Autodesk Inventor part; units mm, degrees
ref_plane "Plano de trabajo1" through (0, 0, 0) normal (0.7071, -0.7071, 0) x (0, 0, 1)
ref_plane "YZ Plane" through (0, 0, 0) normal (1, 0, 0) x (0, 1, 0)
ref_plane "XZ Plane" through (0, 0, 0) normal (0, 1, 0) x (-1, 0, 0)
sketch "Boceto1" plane through (0, 0, 0) normal (0, 0, 1) x (1, 0, 0)
  line L0 (0, 0) -> (0, 25)
  line L1 (0, 0) -> (25, 0)
  line L2 (3, 25) -> (3, 3)
  line L3 (3, 3) -> (25, 3)
  line L4 (0, 25) -> (3, 25)
  line L5 (25, 3) -> (25, 0)
  dimension "d0" = 25
  dimension "d1" = 25
  dimension "d2" = 3
extrude "Extrusión1" add sketch "Boceto1" along normal blind 300
sketch "Boceto2" plane through (0, 0, 0) normal (0, -1, 0) x (1, 0, 0)
  line L0 (0, 0) -> (25, 0) construction
  line L1 (25, 0) -> (25, 300) construction
  line L2 (0, 300) -> (25, 300) construction
  line L3 (0, 0) -> (0, 300) construction
  line L4 (25, 0) -> (25, 300) construction
  line L5 (25, 150) -> (0, 150) construction
  line L6 (25, 300) -> (3, 300)
  line L7 (9, 300) -> (9, 0) construction
  circle A0 centre (9, 159) radius 1.6
  circle A1 centre (9, 141) radius 1.6
  circle A2 centre (9, 279) radius 1.6
  circle A3 centre (9, 261) radius 1.6
  line L8 (25, 270) -> (0, 270) construction
  line L9 (0, 0) -> (0, 300) construction
  dimension "d5" = 3.2
  dimension "d6" = 3.2
  dimension "d7" = 18
  dimension "d8" = 9
  dimension "d9" = 3.2
  dimension "d10" = 3.2
  dimension "d11" = 18
  dimension "d12" = 9
  dimension "d13" = 30
  dimension "d14" = 9
extrude "Extrusión2" cut sketch "Boceto2" against normal through all
ref_plane "Plano de trabajo1" through (0, 0, 0) normal (0.7071, -0.7071, 0) x (0, 0, 1)
mirror "Simetría1" about plane through (0, 0, 0) normal (0.7071, -0.7071, 0) of "Extrusión2"
sketch "Boceto3" plane through (3, 3, 0) normal (0, 1, 0) x (1, 0, 0)
  circle A0 centre (6, -279) radius 1.6 construction
  circle A1 centre (6, -141) radius 1.6 construction
  circle A2 centre (6, -159) radius 1.6 construction
  circle A3 centre (6, -261) radius 1.6 construction
  line L0 (22, 0) -> (0, 0) construction
  line L1 (0, 0) -> (0, -300) construction
  line L2 (22, -300) -> (0, -300) construction
  line L3 (22, 0) -> (22, -300) construction
  circle A4 centre (6, -141) radius 1.6
  circle A5 centre (6, -141) radius 3
  circle A6 centre (6, -159) radius 1.6
  circle A7 centre (6, -159) radius 3
  circle A8 centre (6, -261) radius 1.6
  circle A9 centre (6, -261) radius 3
  circle A10 centre (6, -279) radius 1.6
  circle A11 centre (6, -279) radius 3
  point P0 (-3, 0)
  dimension "d17" = 6
  dimension "d18" = 6
  dimension "d19" = 6
  dimension "d20" = 6
extrude "Extrusión3" cut sketch "Boceto3" against normal blind 2 contours A4 | A5 | A6 | A7 | A8 | A9 | A10 | A11
mirror "Simetría2" about plane through (0, 0, 0) normal (0.7071, -0.7071, 0) of "Extrusión3"
equation "\"d8\" = 0.5 * d7"
equation "\"d12\" = 0.5 * d11"
properties part number "caleta_completa"
Geometry: final body of the model. Coordinates: model frame, mm. A direction names the side the tool comes from. Coordinates: 2 decimals unless noted, no trailing zeros. Order: outer loops, then holes, each group sorted by start corner. A loop starts at its lowest first (then second) coordinate and runs counter-clockwise, first axis right, second up.
1) Draft query along Z for faces 5 (the flat face through (12, 0, 148)), 6 (the flat face through (7, 2, 300)), 7 (the cylindrical face through (2, 9, 282)). Return one class per face: released by +Z, released by -Z, zero draft, split by the parting line, or undercut.
Result sheet:
face 5: zero draft
face 6: released by +Z
face 7: undercut
2) Ray query, probe 1 along Z at (x, y) = (9, 2.3); probe 2 along X at (y, z) = (2, 141); probe 3 along X at (y, z) = (0.5, 279). Return the intervals inside material, ascending.
Result sheet:
probe 1: z = 0 to 138, 144 to 156, 162 to 258, 264 to 276, 282 to 300
probe 2: x = 0 to 6, 12 to 25
probe 3: x = 0 to 7.4, 10.6 to 25
3) Section A-A (z = 209.5). Return loops of the section in (x, y).
Result sheet:
outline: (0, 0) - (25, 0) - (25, 3) - (3, 3) - (3, 25) - (0, 25) - close
4) Section B-B (y = 14.75). Return loops of the section in (x, z).
Result sheet:
outline: (0, 0) - (3, 0) - (3, 300) - (0, 300) - close
5) Set-up query: faces 1 (the flat face through (14, 3, 148)), 2 (the flat face through (7, 2, 0)), 3 (the flat face through (1, 7.7, 160.3)), 4 (the cylindrical face through (10.61, 2.01, 138.47)). Return all of +Z, -Z, +X, -X, +Y, -Y with unobstructed straight access to the full face (end or side cutting, diameter ignored); none if empty.
Result sheet:
face 1: +Z, -Z, +X, +Y
face 2: -Z, +X, -X, +Y, -Y
face 3: +X
face 4: +Y
6) First-contact query: P1, Ø9.5, axis at y = 9, z = 159, coming from the +X side; P2, Ø5.5, axis at x = 9, z = 159, coming from the -Y side; P3, Ø5, axis at x = 9, z = 261, coming from the +Y side; P4, Ø3.5, axis at y = 9, z = 279, coming from the +X side. Flat tips, straight axial feed; report the tip coordinate or a pass-through.
Result sheet:
P1: stops at x = 3
P2: stops at y = 0
P3: stops at y = 1
P4: stops at x = 1
